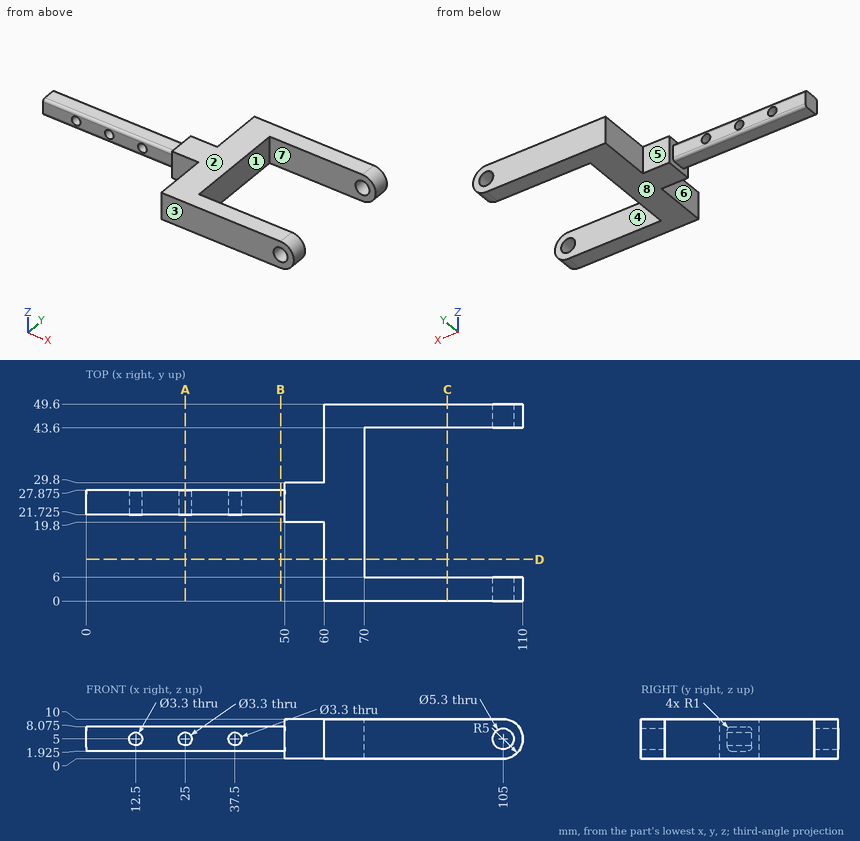
For this review, use the dimensioned drawing (mm, ordinates from the lowest corner) and the shaded views. A direction names the side the tool comes from. Round coordinates to 2 decimals unless told otherwise and drop trailing zeros. Write each loop counter-clockwise with the first axis right and the second up, starting at its lowest first coordinate (ties: lowest second). Pieces come first, ordered by that corner, then holes. Notation, with made-up numbers: (-13.75, 9.25) - (8.25, 9.25) arc R22 ccw to (8.25, 30.25) - close; hole circle Ø8 at (85, 33.25). An arc over 180 degrees is marked (long way). Use a Markdown table: item, result.
Q1. Wall thickness on line 1 along Z through (x, y) = (37.5, 26.5) (3 decimals); line 2 along Y through (x, z) = (89, 5); line 3 along X through (y, z) = (46.7, 5): over which ranges is each line inside the solid? List them lowest first.
Derived:
| item | result |
|---|---|
| line 1 | z = 1.925 to 3.35, 6.65 to 8.075 |
| line 2 | y = 0 to 6, 43.6 to 49.6 |
| line 3 | x = 60 to 102.35, 107.65 to 110 |
Q2. Machinability: for the marked faces 5, 6, 7 and 8, which of the approach directions +Z, -Z, +X, -X, +Y, -Y give a long, thin tool a straight path to every point of the face, cutting with its end or side? Answer none if there is none.
Derived:
| item | result |
|---|---|
| face 5 | +Z, -Z, -X, +Y |
| face 6 | +Z, -Z, -X, -Y |
| face 7 | +Z, -Z, +X |
| face 8 | -Z, +X, -X, +Y, -Y |
Q3. The part is to be moulded in two halves that separate along Y. For the marked faces 1, 2, 3 and 4, say which applies: pulls with the +Y half, pulls with the -Y half, needs draft (parallel to the pull), parting line crosses it, or undercut.
Derived:
| item | result |
|---|---|
| face 1 | undercut |
| face 2 | needs draft |
| face 3 | pulls with the -Y half |
| face 4 | undercut |
Q4. We need section B-B (x = 49). Give the boundary of the cut face in (y, z) (3 decimals), plus the area to 3 significant figures.
Derived:
| item | result |
|---|---|
| outline | (21.725, 2.925) arc R1 ccw to (22.725, 1.925) - (26.875, 1.925) arc R1 ccw to (27.875, 2.925) - (27.875, 7.075) arc R1 ccw to (26.875, 8.075) - (22.725, 8.075) arc R1 ccw to (21.725, 7.075) - close |
| area | 37.0 mm2 |
Q5. Clearance check with flat-ended pins moving along their axes: pin 1 (5.5 mm diameter, centred on x = 12.5, z = 5, fed in from -Y) (3 decimals); pin 2 (3 mm diameter, centred on x = 53, z = 3.5, fed in from -Y); pin 3 (5 mm diameter, centred on y = 23.5, z = 6.5, fed in from -X); pin 4 (2 mm diameter, centred on y = 44, z = 4.5, fed in from -X). State where each tip first meets the part, or that it passes through.
Derived:
| item | result |
|---|---|
| pin 1 | stops at y = 21.725 |
| pin 2 | stops at y = 19.8 |
| pin 3 | stops at x = 0 |
| pin 4 | stops at x = 60 |
Q6. We need section C-C (x = 91). Give the boundary of the cut face in (y, z).
Derived:
| item | result |
|---|---|
| outline | (0, 0) - (6, 0) - (6, 10) - (0, 10) - close; (43.6, 0) - (49.6, 0) - (49.6, 10) - (43.6, 10) - close |
Q7. We need section A-A (x = 25). Give the boundary of the cut face in (y, z) (3 decimals), plus the area to 3 significant figures.
Derived:
| item | result |
|---|---|
| outline | (21.725, 2.925) arc R1 ccw to (22.725, 1.925) - (26.875, 1.925) arc R1 ccw to (27.875, 2.925) - (27.875, 3.35) - (21.725, 3.35) - close; (21.725, 6.65) - (27.875, 6.65) - (27.875, 7.075) arc R1 ccw to (26.875, 8.075) - (22.725, 8.075) arc R1 ccw to (21.725, 7.075) - close |
| area | 16.7 mm2 |
Q8. We need section D-D (y = 10.5). Give the boundary of the cut face in (x, z).
Derived:
| item | result |
|---|---|
| outline | (60, 0) - (70, 0) - (70, 10) - (60, 10) - close |
